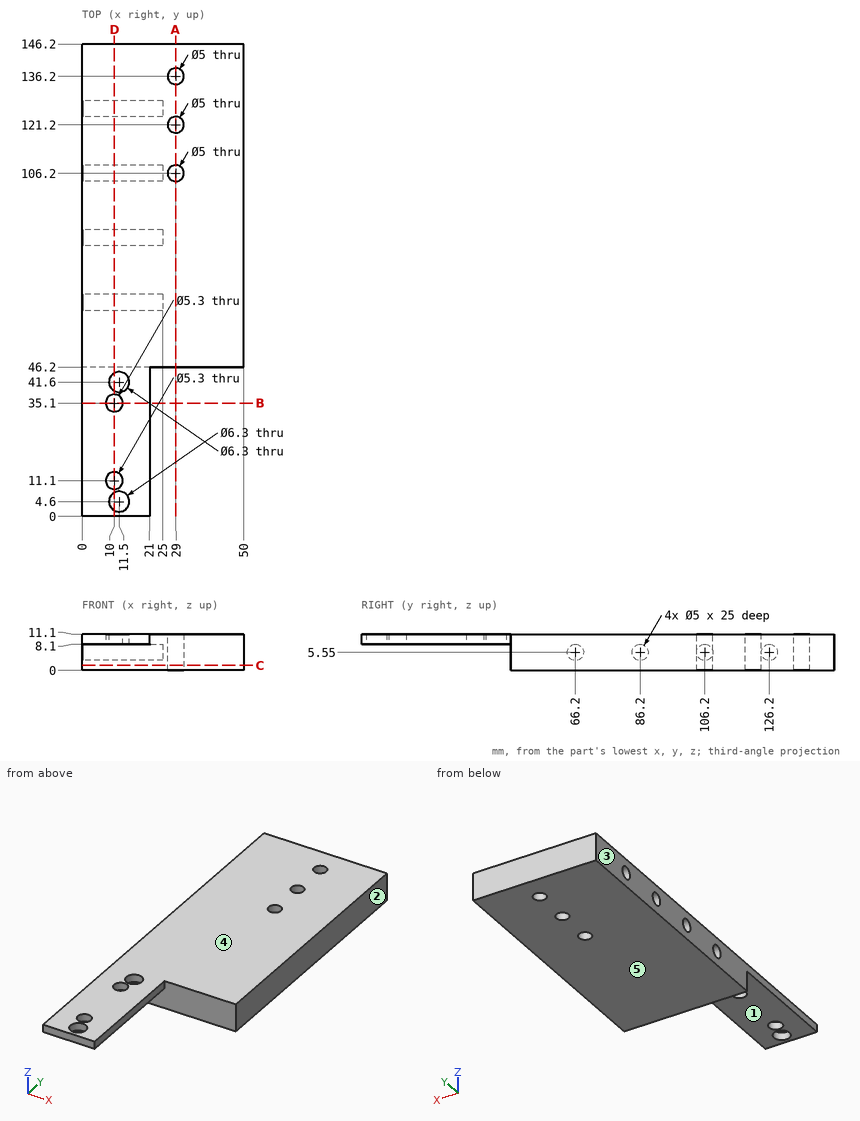
Geometry check sheet. Reference: drawing and pictorial views, mm from the part's lowest x, y, z. A direction names the side the tool comes from. Give positions to 0.01 mm unless a question says otherwise; leave off trailing zeros. Loops run counter-clockwise (first coordinate to the right, second up) from the corner with the lowest first, then second, coordinate; pieces in that order, holes last. Notation, with made-up numbers: (30, 38.25) -> (46, 38.25) arc R36 cw to (46, 73.25) -> close; hole circle Ø11 at (-5.75, -9.5). An arc over 180 degrees is marked (long way). Answer in a Markdown table with one row per item. Add a question column.
1) Gauge pin test, flat ends, axial feed: P1, Ø3.5, axis at y = 32, z = 9.5, coming from the +X side; P2, Ø3.5, axis at x = 29, z = 6, coming from the -Y side; P3, Ø1.5, axis at y = 126, z = 5.5, coming from the -X side; P4, Ø4.5, axis at x = 29, y = 136.2, coming from the -Z side. Record the tip position at first contact, or that the pin passes through.
2) Cross-section at A-A on x = 29. Record the boundary of the cut face in (y, z), and give its area (4 significant figures).
3) Material ranges on probe 1 along Y at (x, z) = (29, 8); probe 2 along Z at (x, y) = (14, 66); probe 3 along X at (y, z) = (121.2, 3), recorded low to high. Write a range as from..to.
4) Set-up check for the marked faces 1 and 2: record each of +Z, -Z, +X, -X, +Y, -Y from which the full face is reachable in a straight line by a thin tool's end or side.
5) Cross-section at B-B on y = 35.1. Record the boundary of the cut face in (x, z).
6) Cross-section at C-C on z = 1.5. Record the boundary of the cut face in (x, y), and give its area (3 significant figures).
7) Draft check along Z on the marked faces 3, 4 and 5. Enter one of: pulls with the +Z half, pulls with the -Z half, needs draft (parallel to the pull), parting line crosses it, or undercut.
8) Cross-section at D-D on x = 10. State how many separate pieces and enclosed holes the cut face has, and give its area (3 significant figures).
Outcome:
| question | item | result |
|---|---|---|
| 1 | P1 | stops at x = 21 |
| 1 | P2 | stops at y = 46.2 |
| 1 | P3 | stops at x = 25 |
| 1 | P4 | passes through |
| 2 | outline | (46.2, 0) -> (103.7, 0) -> (103.7, 11.1) -> (46.2, 11.1) -> close; (108.7, 0) -> (118.7, 0) -> (118.7, 11.1) -> (108.7, 11.1) -> close; (123.7, 0) -> (133.7, 0) -> (133.7, 11.1) -> (123.7, 11.1) -> close; (138.7, 0) -> (146.2, 0) -> (146.2, 11.1) -> (138.7, 11.1) -> close |
| 2 | area | 943.5 mm^2 |
| 3 | probe 1 | y = 46.2..103.7, 108.7..118.7, 123.7..133.7, 138.7..146.2 |
| 3 | probe 2 | z = 0..3.06, 8.04..11.1 |
| 3 | probe 3 | x = 0..26.5, 31.5..50 |
| 4 | face 1 | -Z, +X, -X, -Y |
| 4 | face 2 | +Z, -Z, +X, +Y, -Y |
| 5 | outline | (0, 8.1) -> (7.35, 8.1) -> (7.35, 11.1) -> (0, 11.1) -> close; (12.65, 8.1) -> (21, 8.1) -> (21, 11.1) -> (12.65, 11.1) -> close |
| 6 | outline | (0, 46.2) -> (50, 46.2) -> (50, 146.2) -> (0, 146.2) -> close; hole circle Ø5 at (29, 106.2); hole circle Ø5 at (29, 121.2); hole circle Ø5 at (29, 136.2) |
| 6 | area | 4,940 mm^2 |
| 7 | face 3 | needs draft |
| 7 | face 4 | pulls with the +Z half |
| 7 | face 5 | pulls with the -Z half |
| 8 | separate pieces | 5 |
| 8 | enclosed holes | 4 |
| 8 | area | 1,110 mm^2 |
